Autodesk Inventor part; units mm, degrees
ref_plane "FDT_MOUNT_XY" through (0, 0, 8) normal (0, 0, 1) x (0, 1, 0)
ref_plane "FDT_MOUNT_YZ" through (0, 0, 8) normal (0, 1, 0) x (-1, 0, 0)
ref_plane "FDT_MOUNT_ZX" through (0, 0, 8) normal (-1, 0, 0) x (0, 0, 1)
sketch "Skizze_1" plane through (0, 0, 0) normal (0, 0, 1) x (1, 0, 0)
  line L0 (-18, 35) -> (-18, -35)
  line L1 (-18, -35) -> (18, -35)
  line L2 (18, -35) -> (18, 35)
  line L3 (18, 35) -> (-18, 35)
  circle A0 centre (0, 27.5) radius 3.3
  circle A1 centre (0, -27.5) radius 3.3
extrude "Extrusion1" add sketch "Skizze_1" along normal blind 8
sketch "Skizze_2_ALT_Drilling_1" plane through (0, 0, 0) normal (1, 0, 0) x (0, 1, 0)
  line L0 (0, 0) -> (0, 8)
  line L1 (0, 8) -> (10, 8)
  line L2 (10, 8) -> (9, 7)
  line L3 (9, 7) -> (9, 0)
  line L4 (9, 0) -> (0, 0)
  line L5 (0, 0) -> (0, 8)
revolve "Revolution1" cut sketch "Skizze_2_ALT_Drilling_1" angle 360 about axis through (0, 0, 0) along (0, 0, -1)
sketch "Skizze_3_ALT_Drilling_2" plane through (11, 0, 0) normal (1, 0, 0) x (0, 0, -1)
  line L0 (0, 11) -> (-8, 11)
  line L1 (-8, 11) -> (-8, 13.9)
  line L2 (-8, 13.9) -> (-5, 13.9)
  line L3 (-5, 13.9) -> (-5, 16)
  line L4 (-5, 16) -> (0, 16)
  line L5 (0, 16) -> (0, 11)
  line L6 (0, 11) -> (-8, 11)
revolve "Revolution2" cut sketch "Skizze_3_ALT_Drilling_2" angle 360 about axis through (11, 11, 0) along (0, 0, -1)
sketch "Muster_1_SKETCH_1" plane through (-11, 0, 0) normal (1, 0, 0) x (0, 0, -1)
  line L0 (0, 11) -> (-8, 11)
  line L1 (-8, 11) -> (-8, 13.9)
  line L2 (-8, 13.9) -> (-5, 13.9)
  line L3 (-5, 13.9) -> (-5, 16)
  line L4 (-5, 16) -> (0, 16)
  line L5 (0, 16) -> (0, 11)
  line L6 (0, 11) -> (-8, 11)
sketch "Muster_1_SKETCH_2" plane through (11, 0, 0) normal (1, 0, 0) x (0, 0, -1)
  line L0 (0, -11) -> (-8, -11)
  line L1 (-8, -11) -> (-8, -8.1)
  line L2 (-8, -8.1) -> (-5, -8.1)
  line L3 (-5, -8.1) -> (-5, -6)
  line L4 (-5, -6) -> (0, -6)
  line L5 (0, -6) -> (0, -11)
  line L6 (0, -11) -> (-8, -11)
sketch "Muster_1_SKETCH_3" plane through (-11, 0, 0) normal (1, 0, 0) x (0, 0, -1)
  line L0 (0, -11) -> (-8, -11)
  line L1 (-8, -11) -> (-8, -8.1)
  line L2 (-8, -8.1) -> (-5, -8.1)
  line L3 (-5, -8.1) -> (-5, -6)
  line L4 (-5, -6) -> (0, -6)
  line L5 (0, -6) -> (0, -11)
  line L6 (0, -11) -> (-8, -11)
revolve "Revolution3" cut sketch "Muster_1_SKETCH_1" angle 360 about axis through (-11, 11, 0) along (0, 0, -1)
revolve "Revolution4" cut sketch "Muster_1_SKETCH_2" angle 360 about axis through (11, -11, 0) along (0, 0, -1)
revolve "Revolution5" cut sketch "Muster_1_SKETCH_3" angle 360 about axis through (-11, -11, 0) along (0, 0, -1)
ref_plane "FDT_MOUNT_XY" through (0, 0, 8) normal (0, 0, 1) x (0, 1, 0)
ref_plane "FDT_MOUNT_YZ" through (0, 0, 8) normal (0, 1, 0) x (-1, 0, 0)
ref_plane "FDT_MOUNT_ZX" through (0, 0, 8) normal (-1, 0, 0) x (0, 0, 1)
ref_plane "FNC_1_XY" through (0, 0, 4) normal (0, 0, 1) x (1, 0, 0)
ref_plane "FNC_1_YZ" through (0, 0, 4) normal (1, 0, 0) x (0, 1, 0)
ref_plane "FNC_1_ZX" through (0, 0, 4) normal (0, 1, 0) x (0, 0, 1)
ref_plane "FNC_2_3_XY" through (0, 0, 8) normal (0, 0, 1) x (1, 0, 0)
ref_plane "FNC_2_3_YZ" through (0, 0, 8) normal (1, 0, 0) x (0, 1, 0)
ref_plane "FNC_2_3_ZX" through (0, 0, 8) normal (0, 1, 0) x (0, 0, 1)
ref_plane "FNC_Schraube_1_XY" through (-11, 11, 5) normal (0, 0, 1) x (1, 0, 0)
ref_plane "FNC_Schraube_1_YZ" through (-11, 11, 5) normal (1, 0, 0) x (0, 1, 0)
ref_plane "FNC_Schraube_1_ZX" through (-11, 11, 5) normal (0, 1, 0) x (0, 0, 1)
ref_plane "FNC_Schraube_2_XY" through (11, 11, 5) normal (0, 0, 1) x (1, 0, 0)
ref_plane "FNC_Schraube_2_YZ" through (11, 11, 5) normal (1, 0, 0) x (0, 1, 0)
ref_plane "FNC_Schraube_2_ZX" through (11, 11, 5) normal (0, 1, 0) x (0, 0, 1)
ref_plane "FNC_Schraube_3_XY" through (-11, -11, 5) normal (0, 0, 1) x (1, 0, 0)
ref_plane "FNC_Schraube_3_YZ" through (-11, -11, 5) normal (1, 0, 0) x (0, 1, 0)
ref_plane "FNC_Schraube_3_ZX" through (-11, -11, 5) normal (0, 1, 0) x (0, 0, 1)
ref_plane "FNC_Schraube_4_XY" through (11, -11, 5) normal (0, 0, 1) x (1, 0, 0)
ref_plane "FNC_Schraube_4_YZ" through (11, -11, 5) normal (1, 0, 0) x (0, 1, 0)
ref_plane "FNC_Schraube_4_ZX" through (11, -11, 5) normal (0, 1, 0) x (0, 0, 1)
ref_plane "P17_1_XY" through (0, 27.5, 8) normal (0, 0, 1) x (1, 0, 0)
ref_plane "P17_1_YZ" through (0, 27.5, 8) normal (1, 0, 0) x (0, 1, 0)
ref_plane "P17_1_ZX" through (0, 27.5, 8) normal (0, 1, 0) x (0, 0, 1)
ref_plane "P18_1_XY" through (0, -27.5, 8) normal (0, 0, 1) x (1, 0, 0)
ref_plane "P18_1_YZ" through (0, -27.5, 8) normal (1, 0, 0) x (0, 1, 0)
ref_plane "P18_1_ZX" through (0, -27.5, 8) normal (0, 1, 0) x (0, 0, 1)
properties part number "537247 FNC-20---(F)"
Work out the finished part from the listing and answer in its coordinate system (mm). A direction names the side the tool comes from. Round coordinates to 2 decimals unless told otherwise and drop trailing zeros. Write each loop counter-clockwise with the first axis right and the second up, starting at its lowest first coordinate (ties: lowest second). Pieces come first, ordered by that corner, then holes. Notation, with made-up numbers: (-14.75, -13) - (-2.75, -13) arc R24 cw to (-2.75, 5) - close; hole circle Ø3 at (9.25, 68.5). An arc over 180 degrees is marked (long way). Return JSON: item names as keys, results as strings. Group by question number.
Q1. The mould has two halves that part along Y. Classify faces 3 (the flat face through (-8, 8, 8)), 4 (the flat face through (0, 35, 4)), 5 (the cylindrical face through (-9.5, -6.23, 2.46)): released by +Y, released by -Y, zero draft, split by the parting line, or undercut.
Q2. The part is cut by section A-A on y = 0. Write down the section's boundary in (x, z).
Q3. Each of these flat-tipped pins is pushed along its axis until it touches: pin 1 Ø16 at (x, y) = (11, 11) entering from +Z; pin 2 Ø7.5 at (x, y) = (-11, -11) entering from -Z. Where does it stop, or does it pass through?
Q4. For faces 1 (the cylindrical face through (12.5, -6.23, 2.46)), 2 (the cylindrical face through (-0.72, -24.28, 3.94)), determine the directions among +Z, -Z, +X, -X, +Y, -Y from which every point of the face is accessible in a straight line to the end or side of a thin tool.
Q5. The part is cut by section D-D on y = -11. Write down the section's boundary in (x, z), then the cut area to 3 significant figures.
Q6. The part is cut by section B-B on x = -11. Write down the section's boundary in (y, z).
Q7. Find the intervals of material crossed by L1, parallel to X at y = 11, z = 6.35; L2, parallel to Y at x = 11.5, z = 1; L3, parallel to X at y = 11, z = 4, in increasing order.
Q8. The part is cut by section C-C on z = 3.5. Write down the section's boundary in (x, y), then the cut area to 3 significant figures.
Solved:
{
 "1": {"face 3": "zero draft", "face 4": "released by +Y", "face 5": "undercut"},
 "2": {"outline": "(-18, 0) - (-9, 0) - (-9, 7) - (-10, 8) - (-18, 8) - close; (9, 0) - (18, 0) - (18, 8) - (10, 8) - (9, 7) - close"},
 "3": {"pin 1": "z = 8", "pin 2": "z = 5"},
 "4": {"face 1": "-Z", "face 2": "+Z, -Z"},
 "5": {"outline": "(-18, 0) - (-16, 0) - (-16, 5) - (-13.9, 5) - (-13.9, 8) - (-18, 8) - close; (-8.1, 5) - (-6, 5) - (-6, 0) - (6, 0) - (6, 5) - (8.1, 5) - (8.1, 8) - (-8.1, 8) - close; (13.9, 5) - (16, 5) - (16, 0) - (18, 0) - (18, 8) - (13.9, 8) - close", "area": "153 mm²"},
 "6": {"outline": "(-35, 0) - (-16, 0) - (-16, 5) - (-13.9, 5) - (-13.9, 8) - (-35, 8) - close; (-8.1, 5) - (-6, 5) - (-6, 0) - (6, 0) - (6, 5) - (8.1, 5) - (8.1, 8) - (-8.1, 8) - close; (13.9, 5) - (16, 5) - (16, 0) - (35, 0) - (35, 8) - (13.9, 8) - close"},
 "7": {"L1": "-18 to -13.9, -8.1 to 8.1, 13.9 to 18", "L2": "-35 to -15.97, -6.03 to 6.03, 15.97 to 35", "L3": "-18 to -16, -6 to 6, 16 to 18"},
 "8": {"outline": "(-18, -35) - (18, -35) - (18, 35) - (-18, 35) - close; hole circle Ø10 at (-11, -11); hole circle Ø10 at (-11, 11); hole circle Ø18 at (0, 0); hole circle Ø6.6 at (0, -27.5); hole circle Ø6.6 at (0, 27.5); hole circle Ø10 at (11, -11); hole circle Ø10 at (11, 11)", "area": "1,880 mm²"}
}
